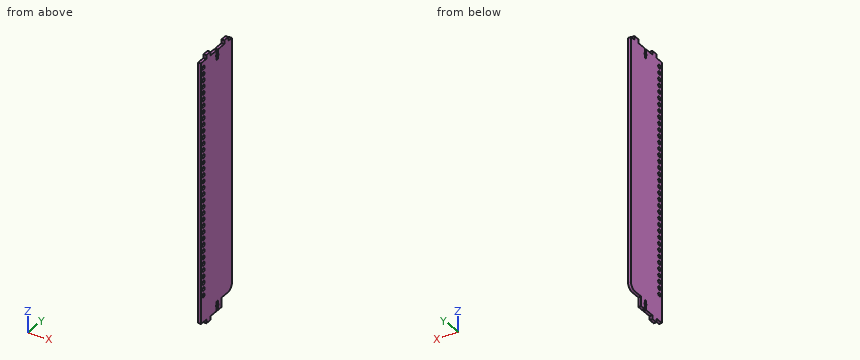
from build123d import *

# Parameters (mm, degrees)
SKETCH1_W           = 412
SKETCH1_H           = 80
BOSS_EXTRUDE1_DEPTH = 4.5
SKETCH4_W           = 4.5
SKETCH4_H           = 10
BOSS_EXTRUDE2_DEPTH = 6
CUT_EXTRUDE3_REACH  = 6.5
SKETCH7_W           = 4.5
SKETCH7_H           = 10
BOSS_EXTRUDE3_DEPTH = 6
SKETCH8_W           = 4.5
SKETCH8_H           = 412
CUT_EXTRUDE4_DEPTH  = 4.5
SKETCH9_W           = 4.5
SKETCH9_H           = 15
CUT_EXTRUDE5_DEPTH  = 25
FILLET1_R           = 10
SKETCH10_R          = 3
CUT_EXTRUDE6_DEPTH  = 4.5


with BuildPart() as part:
    # Sketch1 → Boss-Extrude1 (new body)
    with BuildSketch(Plane(origin=(0, 0, 0), x_dir=(0, 0, -1), z_dir=(1, 0, 0))):
        Rectangle(SKETCH1_W, SKETCH1_H)
    extrude(amount=BOSS_EXTRUDE1_DEPTH)

    # Sketch4 → Boss-Extrude2 (add)
    with BuildSketch(Plane.XY.offset(206)):
        with Locations((2.25, 22)):
            Rectangle(SKETCH4_W, SKETCH4_H)
        with Locations((2.25, -22)):
            Rectangle(SKETCH4_W, SKETCH4_H)
    extrude(amount=BOSS_EXTRUDE2_DEPTH)

    # Sketch5 → Cut-Extrude3 (cut, up to next)
    with BuildSketch(Plane.ZY, mode=Mode.PRIVATE) as cut_extrude3_sk1:
        Polygon((206, -1.6), (206, 1.6), (199, 1.6), (199, 2.8), (196, 2.8), (196, 1.6), (191, 1.6), (191, -1.6), (196, -1.6), (196, -2.8), (199, -2.8), (199, -1.6), align=None)
    cut_extrude3_tool1 = extrude(cut_extrude3_sk1.sketch, amount=-CUT_EXTRUDE3_REACH, mode=Mode.PRIVATE) & part.part
    add(cut_extrude3_tool1.solids().sort_by_distance((0, 0, 198.369565))[0], mode=Mode.SUBTRACT)
    # Sketch5 → Cut-Extrude3 (cut, up to next)
    with BuildSketch(Plane.ZY, mode=Mode.PRIVATE) as cut_extrude3_sk2:
        Polygon((-206, -1.6), (-206, 1.6), (-199, 1.6), (-199, 2.8), (-196, 2.8), (-196, 1.6), (-191, 1.6), (-191, -1.6), (-196, -1.6), (-196, -2.8), (-199, -2.8), (-199, -1.6), align=None)
    cut_extrude3_tool2 = extrude(cut_extrude3_sk2.sketch, amount=-CUT_EXTRUDE3_REACH, mode=Mode.PRIVATE) & part.part
    add(cut_extrude3_tool2.solids().sort_by_distance((0, 0, -198.369565))[0], mode=Mode.SUBTRACT)

    # Sketch7 → Boss-Extrude3 (add)
    with BuildSketch(Plane(origin=(0, 0, -206), x_dir=(-1, 0, 0), z_dir=(0, 0, -1))):
        with Locations((-2.25, -22)):
            Rectangle(SKETCH7_W, SKETCH7_H)
    extrude(amount=BOSS_EXTRUDE3_DEPTH)

    # Sketch8 → Cut-Extrude4 (cut)
    with BuildSketch(Plane(origin=(0, 40, 0), x_dir=(1, 0, 0), z_dir=(0, 1, 0))):
        with Locations((2.25, 0)):
            Rectangle(SKETCH8_W, SKETCH8_H)
    extrude(amount=-CUT_EXTRUDE4_DEPTH, mode=Mode.SUBTRACT)

    # Sketch9 → Cut-Extrude5 (cut)
    with BuildSketch(Plane(origin=(0, 35.5, 0), x_dir=(1, 0, 0), z_dir=(0, 1, 0))):
        with Locations((2.25, 198.5)):
            Rectangle(SKETCH9_W, SKETCH9_H)
    extrude(amount=-CUT_EXTRUDE5_DEPTH, mode=Mode.SUBTRACT)

    # Fillet1
    fillet1_edges = [part.edges().sort_by_distance(p)[0] for p in [
        (2.25, 35.5, -191),
    ]]
    fillet(fillet1_edges, radius=FILLET1_R)

    # Sketch10 → Cut-Extrude6 (cut)
    with BuildSketch(Plane.ZY):
        with Locations((196, -34)):
            Circle(SKETCH10_R)
        with Locations((186, -34)):
            Circle(SKETCH10_R)
        with Locations((176, -34)):
            Circle(SKETCH10_R)
        with Locations((166, -34)):
            Circle(SKETCH10_R)
        with Locations((156, -34)):
            Circle(SKETCH10_R)
        with Locations((146, -34)):
            Circle(SKETCH10_R)
        with Locations((136, -34)):
            Circle(SKETCH10_R)
        with Locations((126, -34)):
            Circle(SKETCH10_R)
        with Locations((116, -34)):
            Circle(SKETCH10_R)
        with Locations((106, -34)):
            Circle(SKETCH10_R)
        with Locations((96, -34)):
            Circle(SKETCH10_R)
        with Locations((86, -34)):
            Circle(SKETCH10_R)
        with Locations((76, -34)):
            Circle(SKETCH10_R)
        with Locations((66, -34)):
            Circle(SKETCH10_R)
        with Locations((56, -34)):
            Circle(SKETCH10_R)
        with Locations((46, -34)):
            Circle(SKETCH10_R)
        with Locations((36, -34)):
            Circle(SKETCH10_R)
        with Locations((26, -34)):
            Circle(SKETCH10_R)
        with Locations((16, -34)):
            Circle(SKETCH10_R)
        with Locations((6, -34)):
            Circle(SKETCH10_R)
        with Locations((-4, -34)):
            Circle(SKETCH10_R)
        with Locations((-14, -34)):
            Circle(SKETCH10_R)
        with Locations((-24, -34)):
            Circle(SKETCH10_R)
        with Locations((-34, -34)):
            Circle(SKETCH10_R)
        with Locations((-44, -34)):
            Circle(SKETCH10_R)
        with Locations((-54, -34)):
            Circle(SKETCH10_R)
        with Locations((-64, -34)):
            Circle(SKETCH10_R)
        with Locations((-74, -34)):
            Circle(SKETCH10_R)
        with Locations((-84, -34)):
            Circle(SKETCH10_R)
        with Locations((-94, -34)):
            Circle(SKETCH10_R)
        with Locations((-104, -34)):
            Circle(SKETCH10_R)
        with Locations((-114, -34)):
            Circle(SKETCH10_R)
        with Locations((-124, -34)):
            Circle(SKETCH10_R)
        with Locations((-134, -34)):
            Circle(SKETCH10_R)
        with Locations((-144, -34)):
            Circle(SKETCH10_R)
        with Locations((-154, -34)):
            Circle(SKETCH10_R)
        with Locations((-164, -34)):
            Circle(SKETCH10_R)
    extrude(amount=-CUT_EXTRUDE6_DEPTH, mode=Mode.SUBTRACT)


solid = part.part
CAD build for the part. Positions are in the model's coordinates, mm. Round coordinates to 2 decimals unless told otherwise and drop trailing zeros. Write each question's results on one line, items separated by ' | '.
1. Cut at A-A (x = 3.1). Count the separate pieces of the cut face and the enclosed holes in it, plus the area to 3 significant figures.
Findings below:
separate pieces: 1 | enclosed holes: 37 | area: 29,700 mm²
2. Flat gauge pins, fed straight in: P1, Ø0.6, axis at x = 1.5, y = -2, coming from the -Z side; P2, Ø1.3, axis at x = 3, y = 18, coming from the -Z side. Where does each tip first touch, or does it go through?
Findings below:
P1: stops at z = -206 | P2: stops at z = -191
3. Wall check: line 1 along Y through (x, z) = (2.1, -34); line 2 along Z through (x, y) = (3.9, 13); line 3 along Z through (x, y) = (0.6, -10). Give the ranges that are in metal, low to high. Write a range as [from, to].
Findings below:
line 1: y = [-40, -37], [-31, 35.5] | line 2: z = [-191, 206] | line 3: z = [-206, 206]
